from build123d import *
from build123d import SkipClean  # not in build123d's __all__

# Parameters (mm, degrees)
F1_DEPTH      = 5
F2_DEPTH      = 10
F2_DEPTH_BACK = 5


with BuildPart() as f1:
    # F0 (on Right) → F1 (new body)
    with BuildSketch(Plane.YZ):
        with BuildLine():
            ThreePointArc((-2.0497591696, 58.6855219415), (-2.7158059717, 67.4442000024), (5, 63.2460578033))
            ThreePointArc((5, 63.2460578033), (4.1565190701, 60.4669663655), (1.9106603122, 58.6255191798))
            Line((1.9106603122, 58.6255191798), (2.6749244371, 56.7773037304))
            ThreePointArc((2.6749244371, 56.7773037304), (5.8191266982, 59.3553297904), (7, 63.2460578033))
            ThreePointArc((7, 63.2460578033), (3.3734494014, 69.3795591799), (-3.7485254675, 69.1577882453))
            ThreePointArc((-3.7485254675, 69.1577882453), (-6.1768933492, 66.539382651), (-6.9976278698, 63.0638376186))
            ThreePointArc((-6.9976278698, 63.0638376186), (-5.827409471, 59.3677464624), (-2.8696628374, 56.8613075968))
            Line((-2.8696628374, 56.8613075968), (-2.0497591696, 58.6855219415))
        make_face()
        with BuildLine():
            ThreePointArc((1.9106603122, 58.6255191798), (-0.0757443456, 58.2466315568), (-2.0497591696, 58.6855219415))
            Line((-2.0497591696, 58.6855219415), (-2.8696628374, 56.8613075968))
            ThreePointArc((-2.8696628374, 56.8613075968), (-2.6859296062, 56.7818654987), (-2.5, 56.707709388))
            Line((-2.5, 56.707709388), (2.5, 56.707709388))
            ThreePointArc((2.5, 56.707709388), (2.5876961907, 56.7419184733), (2.6749244371, 56.7773037304))
            Line((2.6749244371, 56.7773037304), (1.9106603122, 58.6255191798))
        make_face()
        with BuildLine():
            Line((-21.3842253571, 70.7343179555), (-6.9976278698, 63.0638376186))
            ThreePointArc((-6.9976278698, 63.0638376186), (-6.1768933492, 66.539382651), (-3.7485254675, 69.1577882453))
            Line((-3.7485254675, 69.1577882453), (-18.1351229548, 76.8282685822))
            ThreePointArc((-18.1351229548, 76.8282685822), (-17.1255151434, 75.5992014909), (-16.7640988794, 74.0502366327))
            ThreePointArc((-16.7640988794, 74.0502366327), (-18.2233199438, 71.2067842705), (-21.3842253571, 70.7343179555))
        make_face()
        with BuildLine():
            Line((2.5, 56.707709388), (-2.5, 56.707709388))
            ThreePointArc((-2.5, 56.707709388), (0, 56.2460578033), (2.5, 56.707709388))
        make_face()
        with BuildLine():
            ThreePointArc((2.5, 56.707709388), (0, 56.2460578033), (-2.5, 56.707709388))
            Line((-2.5, 56.707709388), (-2.5, 5.6896996604))
            ThreePointArc((-2.5, 5.6896996604), (0, 5.6354306355), (2.5, 5.6896996604))
            Line((2.5, 5.6896996604), (2.5, 56.707709388))
        make_face()
        with BuildLine():
            Line((-20.412130709, 72.5575589791), (-21.3842253571, 70.7343179555))
            ThreePointArc((-21.3842253571, 70.7343179555), (-18.2233199438, 71.2067842705), (-16.7640988794, 74.0502366327))
            ThreePointArc((-16.7640988794, 74.0502366327), (-17.1255151434, 75.5992014909), (-18.1351229548, 76.8282685822))
            Line((-18.1351229548, 76.8282685822), (-19.1072176029, 75.0050275585))
            ThreePointArc((-19.1072176029, 75.0050275585), (-18.8524824452, 74.5575225901), (-18.7640988794, 74.0502366327))
            ThreePointArc((-18.7640988794, 74.0502366327), (-19.2571350629, 72.9384705277), (-20.412130709, 72.5575589791))
        make_face()
        with BuildLine():
            ThreePointArc((-18.1351229548, 76.8282685822), (-23.352545554, 75.6968990565), (-21.3842253571, 70.7343179555))
            Line((-21.3842253571, 70.7343179555), (-20.412130709, 72.5575589791))
            ThreePointArc((-20.412130709, 72.5575589791), (-21.5877188828, 74.7559491), (-19.1072176029, 75.0050275585))
            Line((-19.1072176029, 75.0050275585), (-18.1351229548, 76.8282685822))
        make_face()
        with BuildLine():
            ThreePointArc((2.5, 5.6896996604), (0, 5.6354306355), (-2.5, 5.6896996604))
            ThreePointArc((-2.5, 5.6896996604), (-12.3544556578, 6.9757122555), (-21.8412756578, 9.9361802916))
            ThreePointArc((-21.8412756578, 9.9361802916), (-23.3409375081, 9.9429800309), (-24.4237277351, 8.9053879982))
            Line((-24.4237277351, 8.9053879982), (-25.6964663445, 6.0736552965))
            ThreePointArc((-25.6964663445, 6.0736552965), (-25.7303627866, 4.5138703516), (-24.6335625617, 3.4043175994))
            ThreePointArc((-24.6335625617, 3.4043175994), (-0.9803374174, -1.4600872963), (22.8093950074, 2.6855279633))
            ThreePointArc((22.8093950074, 2.6855279633), (23.939304908, 3.7613447039), (23.9526765567, 5.3214406119))
            Line((23.9526765567, 5.3214406119), (22.7663073553, 8.1904302912))
            ThreePointArc((22.7663073553, 8.1904302912), (21.7154471881, 9.260348424), (20.2162676541, 9.2989829539))
            ThreePointArc((20.2162676541, 9.2989829539), (11.5006058756, 6.7950132854), (2.5, 5.6896996604))
        make_face()
    extrude(amount=F1_DEPTH)

    # F0 (on Right) → F2 (join, two sides)
    with BuildSketch(Plane.YZ) as f2_sk:
        with BuildLine():
            ThreePointArc((1.9106603122, 58.6255191798), (-0.0757443456, 58.2466315568), (-2.0497591696, 58.6855219415))
            Line((-2.0497591696, 58.6855219415), (-2.8696628374, 56.8613075968))
            ThreePointArc((-2.8696628374, 56.8613075968), (-2.6859296062, 56.7818654987), (-2.5, 56.707709388))
            Line((-2.5, 56.707709388), (2.5, 56.707709388))
            ThreePointArc((2.5, 56.707709388), (2.5876961907, 56.7419184733), (2.6749244371, 56.7773037304))
            Line((2.6749244371, 56.7773037304), (1.9106603122, 58.6255191798))
        make_face()
        with BuildLine():
            ThreePointArc((-2.0497591696, 58.6855219415), (-2.7158059717, 67.4442000024), (5, 63.2460578033))
            ThreePointArc((5, 63.2460578033), (4.1565190701, 60.4669663655), (1.9106603122, 58.6255191798))
            Line((1.9106603122, 58.6255191798), (2.6749244371, 56.7773037304))
            ThreePointArc((2.6749244371, 56.7773037304), (5.8191266982, 59.3553297904), (7, 63.2460578033))
            ThreePointArc((7, 63.2460578033), (3.3734494014, 69.3795591799), (-3.7485254675, 69.1577882453))
            ThreePointArc((-3.7485254675, 69.1577882453), (-6.1768933492, 66.539382651), (-6.9976278698, 63.0638376186))
            ThreePointArc((-6.9976278698, 63.0638376186), (-5.827409471, 59.3677464624), (-2.8696628374, 56.8613075968))
            Line((-2.8696628374, 56.8613075968), (-2.0497591696, 58.6855219415))
        make_face()
        with BuildLine():
            Line((2.5, 56.707709388), (-2.5, 56.707709388))
            ThreePointArc((-2.5, 56.707709388), (0, 56.2460578033), (2.5, 56.707709388))
        make_face()
    with SkipClean():  # cleaning this boolean's faces spoils the solid; the shape is the same uncleaned
        extrude(amount=F2_DEPTH)
        extrude(f2_sk.sketch, amount=-F2_DEPTH_BACK)


solid = f1.part
Design review of the part built by this model. Coordinates are the model's own, in mm. A direction names the side the tool comes from. Give positions to 0.01 mm unless a question says otherwise; leave off trailing zeros. Order: outer loops, then holes, each group sorted by start corner. A loop starts at its lowest first (then second) coordinate and runs counter-clockwise, first axis right, second up.
1. For pin 1 Ø1.8 at (y, z) = (-20.26, 74.05) entering from +X; pin 2 Ø8 at (x, z) = (1, 65.5) entering from +Y; pin 3 Ø1.5 at (x, z) = (2, 41.5) entering from -Y; pin 4 Ø6 at (x, y) = (0.5, -11.5) entering from -Z, all flat-tipped, find the tip position at first contact; note any pin that passes through.
Solution:
pin 1: passes through
pin 2: stops at y = 7
pin 3: stops at y = -2.5
pin 4: stops at z = -0.91
2. Add section A-A, the plane x = 1.25. State the section outline as (y, z) points.
Solution:
outline: (-25.7, 6.07) arc R2 ccw to (-24.63, 3.4) arc R64.71 ccw to (22.81, 2.69) arc R2 ccw to (23.95, 5.32) - (22.77, 8.19) arc R2 ccw to (20.22, 9.3) arc R57.61 cw to (2.5, 5.69) - (2.5, 56.71) arc R7 ccw (long way) to (-3.75, 69.16) - (-18.14, 76.83) arc R3.5 ccw (long way) to (-21.38, 70.73) - (-7, 63.06) arc R7 ccw to (-2.5, 56.71) - (-2.5, 5.69) arc R57.61 cw to (-21.84, 9.94) arc R2 ccw to (-24.42, 8.91) - close; hole circle Ø3 at (-20.26, 74.05); hole circle Ø10 at (0, 63.25)
3. Tool access review of faces 1 (the cylindrical face through (2.465, -12.218, 6.946)), 2 (the flat face through (5, -1, 15)), 3 (the flat face through (10, -5, 65)), 4 (the flat face through (0, -1, 15)), 5 (the flat face through (2.46, -14.29, 66.95)): name each direction out of +Z, -Z, +X, -X, +Y, -Y from which nothing blocks a thin tool from reaching the whole face with its end or side.
Solution:
face 1: +X, -X
face 2: -Z, +X, +Y, -Y
face 3: +Z, -Z, +X, +Y, -Y
face 4: -Z, -X, +Y, -Y
face 5: +X, -X, -Y
4. Add section B-B, the plane y = 0. State the section outline as (x, z) points, then the cut area to 3 significant figures.
Solution:
outline: (-5, 56.25) - (0, 56.25) - (0, -1.47) - (5, -1.47) - (5, 56.25) - (10, 56.25) - (10, 58.25) - (-5, 58.25) - close; (-5, 68.25) - (10, 68.25) - (10, 70.25) - (-5, 70.25) - close
area: 349 mm2
5. Add section C-C, the plane x = -3.5. State the section outline as (y, z) points.
Solution:
outline: circle Ø14 at (0, 63.25); hole circle Ø10 at (0, 63.25)
6. Add section D-D, the plane y = -10.5. State the section outline as (x, z) points, then the cut area to 3 significant figures.
Solution:
outline: (0, -0.61) - (5, -0.61) - (5, 6.6) - (0, 6.6) - close; (0, 64.93) - (5, 64.93) - (5, 72.76) - (0, 72.76) - close
area: 75.2 mm2
7. Mouldability with a two-part tool opening along Y and no side actions: class faces 6 (the cylindrical face through (2.46, 23.93, 3.74)), 7 (the flat face through (-5, -5, 65)), 8 (the cylindrical face through (2.46, -23.32, 9.95)) as +Y half, -Y half, draft (parallel to the pull), parting line (faces both ways), or undercut.
Solution:
face 6: +Y half
face 7: draft
face 8: undercut
8. To check wall thickness, follow L1, parallel to X at y = 13.5, z = 3; L2, parallel to Z at x = 2.25, y = -7.5; L3, parallel to Z at x = 1.5, y = -5.5. State the ranges of each line that lie inside material, in increasing order.
Solution:
L1: x = 0 to 5
L2: z = -1.03 to 6.13, 63.33 to 71.16
L3: z = -1.23 to 5.9, 58.92 to 70.09
